```python
from build123d import *

# Parameters (mm, degrees)
F1_DEPTH = 25.4


with BuildPart() as f1:
    # F0 (on Front) → F1 (new body)
    with BuildSketch(Plane.XZ):
        with BuildLine():
            ThreePointArc((-113.665045, -18.445694), (-91.184621, -13.32064), (-81.178721, 7.452363))
            ThreePointArc((-81.178721, 7.452363), (-88.835816, 26.112679), (-107.393124, 34.016147))
            ThreePointArc((-107.393124, 34.016147), (-134.123105, 10.60594), (-113.665045, -18.445694))
        make_face()
        with BuildLine():
            ThreePointArc((-107.393124, 34.016147), (-88.835816, 26.112679), (-81.178721, 7.452363))
            ThreePointArc((-81.178721, 7.452363), (-91.184621, -13.32064), (-113.665045, -18.445694))
            Line((-113.665045, -18.445694), (-53.619757, -32.171853))
            Line((-53.619757, -32.171853), (-53.619757, 33.205918))
            Line((-53.619757, 33.205918), (-46.198466, 33.205918))
            Line((-46.198466, 33.205918), (-107.393124, 34.016147))
        make_face()
        Polygon((28.628288, 33.205918), (-46.198466, 33.205918), (-53.619757, 33.205918), (-53.619757, -32.171853), (28.628288, -32.171853), align=None)
        with BuildLine():
            Line((61.43455, 14.125688), (28.628288, 33.205918))
            Line((28.628288, 33.205918), (28.628288, -32.171853))
            Line((28.628288, -32.171853), (62.983333, -2.468457))
            ThreePointArc((62.983333, -2.468457), (46.094147, 4.324571), (61.43455, 14.125688))
        make_face()
        with BuildLine():
            ThreePointArc((66.525181, 5.27595), (65.161731, 10.380663), (61.43455, 14.125688))
            ThreePointArc((61.43455, 14.125688), (46.094147, 4.324571), (62.983333, -2.468457))
            ThreePointArc((62.983333, -2.468457), (65.597707, 1.018), (66.525181, 5.27595))
        make_face()
    extrude(amount=F1_DEPTH)


solid = f1.part
```
Geometry check sheet. Reference: the model listing, model coordinates, mm. A direction names the side the tool comes from. Give positions to 0.01 mm unless a question says otherwise; leave off trailing zeros. Loops run counter-clockwise (first coordinate to the right, second up) from the corner with the lowest first, then second, coordinate; pieces in that order, holes last. Notation, with made-up numbers: M 39,-21.5 L 91,-21.5 A20 cw 91,-11.5 Z; hole C 43.25,36 d6. An arc over 180 degrees is marked long. Answer as CSV lines item,"result".
Item 1: Cross-section at A-A on y = -22. Record the cut outline in (x, z).
Values:
outline,"M -113.67,-18.45 L -53.62,-32.17 L 28.63,-32.17 L 62.98,-2.47 A10.24 ccw 66.53,5.28 A10.24 ccw 61.43,14.13 L 28.63,33.21 L -46.2,33.21 L -107.39,34.02 A26.57 ccw Z"
Item 2: Material ranges on line 1 (Z direction, x = -47, y = -8); line 2 (X direction, y = -8.25, z = -5.5); line 3 (X direction, y = -1.75, z = -6.5), recorded low to high.
Values:
line 1,"z = -32.17 to 33.22"
line 2,"x = -130.94 to 59.48"
line 3,"x = -130.35 to 58.32"
Item 3: Depth check by flat-ended pin: P1, Ø3, axis at y = -10.5, z = 23, coming from the -X side; P2, Ø8, axis at x = -112.5, y = -19, coming from the +Z side; P3, Ø2, axis at y = -3.5, z = 20.5, coming from the -X side. Enter the tip coordinate at first touch or a pass-through.
Values:
P1,"stops at x = -130.29"
P2,"stops at z = 34.01"
P3,"stops at x = -131.42"
Item 4: Cross-section at B-B on z = -22. Record the cut outline in (x, y).
Values:
outline,"M -98.12,-25.4 L 40.39,-25.4 L 40.39,0 L -98.12,0 Z"
Item 5: Cross-section at C-C on x = -60.5. Record the cut outline in (y, z).
Values:
outline,"M -25.4,-30.6 L 0,-30.6 L 0,33.4 L -25.4,33.4 Z"
Item 6: Access from +Z, -Z, +X, -X, +Y, -Y to the whole of each face (thin tool, end or side, straight path). Record for faces 1 (the flat face through (-8, -13, 33.206)), 2 (the flat face through (45.6, -12.5, -17.5)).
Values:
face 1,"+Z, +X, +Y, -Y"
face 2,"-Z, +X, +Y, -Y"
